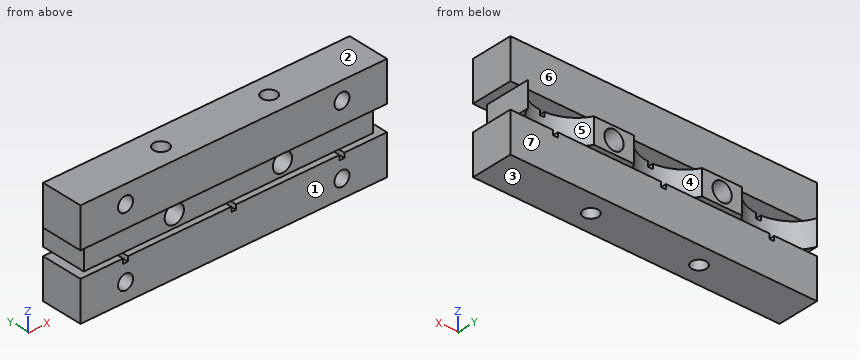
from build123d import *

# Parameters (mm, degrees)
BOSS_EXTRUDE1_DEPTH              = 4.2
SKETCH3_R                        = 1.6
CUT_EXTRUDE3_DEPTH               = 26.650611325
LPATTERN1_COUNT                  = 2
LPATTERN1_PITCH                  = 18
SKETCH6_W                        = 51
SKETCH6_H                        = 7
BOSS_EXTRUDE3_DEPTH              = 6.65
SKETCH7_W                        = 0.8
SKETCH7_H                        = 0.8
CUT_EXTRUDE7_DEPTH               = 28.734190536
SKETCH8_W                        = 51
SKETCH8_H                        = 7
BOSS_EXTRUDE4_DEPTH              = 6.65
TAP_DRILL_FOR_M3_TAP1_AT_2_COUNT = 2
TAP_DRILL_FOR_M3_TAP1_AT_2_PITCH = 18
LPATTERN2_COUNT                  = 2
LPATTERN2_PITCH                  = 36
LPATTERN2_COUNT_DIR2             = 2
LPATTERN2_PITCH_DIR2             = 11.5
SKETCH16_W                       = 48.12122682
SKETCH16_H                       = 4.2
CUT_EXTRUDE8_DEPTH               = 1


with BuildPart() as part:
    # Sketch1 → Boss-Extrude1 (new body)
    with BuildSketch(Plane.XY):
        with BuildLine():
            Line((-12.324882265, -9.164137338), (-5.677872392, -9.164137338))
            ThreePointArc((-5.677872392, -9.164137338), (0, -12.5), (5.677872392, -9.164137338))
            Line((5.677872392, -9.164137338), (12.324882265, -9.164137338))
            ThreePointArc((12.324882265, -9.164137338), (18.449107388, -12.484656447), (24.06061341, -8.356341939))
            Line((24.06061341, -8.356341939), (24.06061341, -17))
            Line((24.06061341, -17), (-24.06061341, -17))
            Line((-24.06061341, -17), (-24.06061341, -8.356341939))
            ThreePointArc((-24.06061341, -8.356341939), (-18.449107388, -12.484656447), (-12.324882265, -9.164137338))
        make_face()
    extrude(amount=BOSS_EXTRUDE1_DEPTH)

    # Sketch3 → Cut-Extrude3 (cut, through all)
    with BuildSketch(Plane(origin=(0, -9.164137338, 0), x_dir=(1, 0, 0), z_dir=(0, 1, 0))):
        with Locations(Location((-9.001377329, -2.1, 0), (0, 0, 270))):
            Circle(SKETCH3_R)
    cut_extrude3 = extrude(amount=-CUT_EXTRUDE3_DEPTH, mode=Mode.SUBTRACT)

    # LPattern1: Cut-Extrude3 ×2
    with Locations(*[(i * LPATTERN1_PITCH, 0, 0) for i in range(1, LPATTERN1_COUNT)]):
        add(cut_extrude3, mode=Mode.SUBTRACT)

    # Sketch6 → Boss-Extrude3 (add)
    with BuildSketch(Plane(origin=(0, 0, 0), x_dir=(-1, 0, 0), z_dir=(0, 0, -1))):
        with Locations((0, -13.5)):
            Rectangle(SKETCH6_W, SKETCH6_H)
    extrude(amount=BOSS_EXTRUDE3_DEPTH)

    # Sketch7 → Cut-Extrude7 (cut, through all)
    with BuildSketch(Plane.XZ.offset(17)):
        with Locations((-0.002754658, 3.8)):
            Rectangle(SKETCH7_W, SKETCH7_H)
        with Locations((-18.002754658, -0.4)):
            Rectangle(SKETCH7_W, SKETCH7_H)
        with Locations((-18.002754658, 3.8)):
            Rectangle(SKETCH7_W, SKETCH7_H)
        with Locations((-0.002754658, -0.4)):
            Rectangle(SKETCH7_W, SKETCH7_H)
        with Locations((17.997245342, 3.8)):
            Rectangle(SKETCH7_W, SKETCH7_H)
        with Locations((17.997245342, -0.4)):
            Rectangle(SKETCH7_W, SKETCH7_H)
    extrude(amount=-CUT_EXTRUDE7_DEPTH, mode=Mode.SUBTRACT)

    # Sketch8 → Boss-Extrude4 (add)
    with BuildSketch(Plane.XY.offset(4.2)):
        with Locations((0, -13.5)):
            Rectangle(SKETCH8_W, SKETCH8_H)
    extrude(amount=BOSS_EXTRUDE4_DEPTH)

    # Sketch13 → Tap Drill for M3 Tap1 (revolve, cut)
    with BuildSketch(Plane(origin=(9, -13.5, -6.65), x_dir=(0, 1, 0), z_dir=(1, 0, 0))):
        Polygon((0, 0), (0, 6.751075774), (1.25, 6), (1.25, 0), align=None)
    tap_drill_for_m3_tap1 = revolve(axis=Axis((9, -13.5, -13), (0, 0, 1)), mode=Mode.SUBTRACT)

    # Tap Drill for M3 Tap1 at 2: Tap Drill for M3 Tap1 ×2
    with Locations(*[(-i * TAP_DRILL_FOR_M3_TAP1_AT_2_PITCH, 0, 0) for i in range(1, TAP_DRILL_FOR_M3_TAP1_AT_2_COUNT)]):
        add(tap_drill_for_m3_tap1, mode=Mode.SUBTRACT)

    # Mirror2: Tap Drill for M3 Tap1 across plane
    add(tap_drill_for_m3_tap1.mirror(Plane.XY.offset(2.1)), mode=Mode.SUBTRACT)

    # Mirror2 copy 1 sketch → Mirror2 copy 1 (revolve, cut)
    with BuildSketch(Plane(origin=(-9, -13.5, 10.85), x_dir=(0, 1, 0), z_dir=(1, 0, 0))):
        Polygon((0, 0), (0, -6.751075774), (1.25, -6), (1.25, 0), align=None)
    revolve(axis=Axis((-9, -13.5, 17.2), (0, 0, 1)), mode=Mode.SUBTRACT)

    # Sketch15 → M3 Tapped Hole3 (revolve, cut)
    with BuildSketch(Plane(origin=(-18, -17, 7.85), x_dir=(0, 0, -1), z_dir=(1, 0, 0))):
        Polygon((0, 0), (0, 6.251075774), (1.25, 5.5), (1.25, 0), align=None)
    m3_tapped_hole3 = revolve(axis=Axis((-18, -23.35, 7.85), (0, 1, 0)), mode=Mode.SUBTRACT)

    # LPattern2: M3 Tapped Hole3 2 × 2
    with Locations(*[(i * LPATTERN2_PITCH, 0, -j * LPATTERN2_PITCH_DIR2) for i in range(LPATTERN2_COUNT) for j in range(LPATTERN2_COUNT_DIR2) if (i, j) != (0, 0)]):
        add(m3_tapped_hole3, mode=Mode.SUBTRACT)

    # Sketch16 → Cut-Extrude8 (cut)
    with BuildSketch(Plane.XZ.offset(17)):
        with Locations((0, 2.1)):
            Rectangle(SKETCH16_W, SKETCH16_H)
    extrude(amount=-CUT_EXTRUDE8_DEPTH, mode=Mode.SUBTRACT)


solid = part.part
The model under review builds one solid part; all positions refer to its coordinate system, in mm. Face numbers are marked on the shaded views. A direction names the side the tool comes from. Give positions to 0.01 mm unless a question says otherwise; leave off trailing zeros. Order: outer loops, then holes, each group sorted by start corner. A loop starts at its lowest first (then second) coordinate and runs counter-clockwise, first axis right, second up. Notation, with made-up numbers: M 35,-34.75 L 82,-34.75 A37 cw 82,4.25 Z; hole C 68.5,-10 d6. An arc over 180 degrees is marked long. Use one line per item in the form item = value. Start each with the question number.
Item 1: To check wall thickness, follow line 1 along Z through (x, y) = (18, -13.3); line 2 along Z through (x, y) = (-19.5, -16.5); line 3 along X through (y, z) = (-14.25, -0.75). State the ranges of each line that lie inside material, in increasing order. Write a range as from..to.
Item 2: We need section A-A on z = 2.1. Give the boundary of the cut face in (x, y).
Item 3: We need section C-C on z = -3. Give the number of separate pieces and of enclosed holes in the cut face, plus the area to 3 significant figures.
Item 4: We need section B-B on x = -15.5. Give the boundary of the cut face in (y, z), plus the area to 3 significant figures.
Item 5: For the marked faces 5, 6 and 7, list the 3-axis set-ups (+Z, -Z, +X, -X, +Y, -Y) from which the entire face can be reached by the end or side of a thin tool; tool diameter is ignored.
Item 6: The part is to be moulded in two halves that separate along Z. For the marked faces 1, 2, 3 and 4, say which applies: pulls with the +Z half, pulls with the -Z half, needs draft (parallel to the pull), parting line crosses it, or undercut.
Item 7: Insertion check: pin 1 Ø2 at (x, z) = (19.5, 5) entering from +Y; pin 2 Ø4.5 at (x, z) = (10, 1.5) entering from +Y; pin 3 Ø3 at (x, z) = (6.5, 2.5) entering from -Y; pin 4 Ø2.5 at (x, z) = (9, 2.1) entering from -Y. Each pin has a flat end and moves straight along its axis. Give the tip position at first contact, or say it passes through.
Completed:
q1.line_1 = -6.65..-4.9, -2.4..-0.8, 0..3.4, 4.2..6.6, 9.1..10.85
q1.line_2 = -6.65..0, 4.2..10.85
q1.line_3 = -25.5..-18.4, -17.6..-10, -8..-0.4, 0.4..8, 10..17.6, 18.4..25.5
q2.outline = M -24.06,-16 L -10.6,-16 L -10.6,-9.16 L -12.32,-9.16 A6.5 cw -24.06,-8.36 Z; M -7.4,-16 L 7.4,-16 L 7.4,-9.16 L 5.68,-9.16 A6.5 cw -5.68,-9.16 L -7.4,-9.16 Z; M 10.6,-16 L 24.06,-16 L 24.06,-8.36 A6.5 cw 12.32,-9.16 L 10.6,-9.16 Z
q3.separate_pieces = 1
q3.enclosed_holes = 2
q3.area = 323 mm²
q4.outline = M -17,-6.65 L -10,-6.65 L -10,0 L -12,0 L -12,4.2 L -10,4.2 L -10,10.85 L -17,10.85 L -17,4.2 L -16,4.2 L -16,0 L -17,0 Z
q4.area = 110 mm²
q5.face_5 = +Y
q5.face_6 = +Z, +X, -X, +Y
q5.face_7 = -Z, +X, -X, +Y
q6.face_1 = needs draft
q6.face_2 = pulls with the +Z half
q6.face_3 = pulls with the -Z half
q6.face_4 = undercut
q7.pin_1 = -10
q7.pin_2 = -9.16
q7.pin_3 = -16
q7.pin_4 = through
